from build123d import *

# Parameters (mm, degrees)
SKETCH1_W               = 155
SKETCH1_H               = 163
BOSS_EXTRUDE1_DEPTH     = 10
SKETCH2_R               = 1.5
CUT_EXTRUDE1_DEPTH      = 20
CUT_EXTRUDE2_DEPTH      = 226.153281122
CUT_EXTRUDE2_DEPTH_BACK = 226.153281122
SKETCH3_R               = 1.5


with BuildPart() as part:
    # Sketch1 → Boss-Extrude1 (new body)
    with BuildSketch(Plane(origin=(0, 0, 0), x_dir=(1, 0, 0), z_dir=(0, 1, 0))):
        with Locations((77.5, 81.5)):
            Rectangle(SKETCH1_W, SKETCH1_H)
    extrude(amount=BOSS_EXTRUDE1_DEPTH)

    # Sketch2 → Cut-Extrude1 (cut)
    with BuildSketch(Plane(origin=(0, 0, -163), x_dir=(-1, 0, 0), z_dir=(0, 0, -1))):
        with Locations((-125, 5)):
            Circle(SKETCH2_R)
        with Locations(Location((-30, 5, 0), (0, 0, 180))):
            Circle(SKETCH2_R)
    cut_extrude1 = extrude(amount=-CUT_EXTRUDE1_DEPTH, mode=Mode.SUBTRACT)

    # Mirror1: Cut-Extrude1 across plane
    add(cut_extrude1.mirror(Plane(origin=(0, 0, -81.5), x_dir=(1, 0, 0), z_dir=(0, 0, -1))), mode=Mode.SUBTRACT)

    # Sketch3 → Cut-Extrude2 (cut, two sides: drawn at the far end of the back side and taken through both)
    with BuildSketch(Plane(origin=(155, 0, 0), x_dir=(0, 0, -1), z_dir=(1, 0, 0)).offset(-CUT_EXTRUDE2_DEPTH_BACK)):
        with Locations((35, 5)):
            Circle(SKETCH3_R)
        with Locations(Location((128, 5, 0), (0, 0, 180))):
            Circle(SKETCH3_R)
    extrude(amount=CUT_EXTRUDE2_DEPTH + CUT_EXTRUDE2_DEPTH_BACK, mode=Mode.SUBTRACT)


solid = part.part
The listing builds one solid part. Answer for the finished solid, in the listing's coordinates (mm). Coordinates: 2 decimals unless noted, no trailing zeros. Write each loop counter-clockwise with the first axis right and the second up, starting at its lowest first coordinate (ties: lowest second). Pieces come first, ordered by that corner, then holes. Notation, with made-up numbers: (63.25, 55) - (80.25, 55) arc R20 ccw to (80.25, 61) - close; hole circle Ø3 at (-11.5, -19). An arc over 180 degrees is marked (long way). Return JSON: item names as keys, results as strings.
1. For a pull along X with two mould halves and no side action, classify faces 1 (the face through (76, 5, 0)), 2 (the face through (0, 5, -80)), 3 (the face through (155, 5, -80)) as +X half, -X half, draft (parallel to the pull), parting line (faces both ways), or undercut.
Final values:
{"face 1": "draft", "face 2": "-X half", "face 3": "+X half"}
2. Consider line 1 along Z through (x, y) = (142.5, 4.75); line 2 along Y through (x, z) = (30, -149.5); line 3 along Z through (x, y) = (20, 6.25). Determine where each line is inside the solid, lowest interval first.
Final values:
{"line 1": "-163 to -129.48, -126.52 to -36.48, -33.52 to 0", "line 2": "0 to 3.5, 6.5 to 10", "line 3": "-163 to -128.83, -127.17 to -35.83, -34.17 to 0"}
3. The part is cut by section A-A on y = 5. Determine the outline of the cut face in (x, z), then the cut area to 3 significant figures.
Final values:
{"outline": "(0, -163) - (28.5, -163) - (28.5, -143) - (31.5, -143) - (31.5, -163) - (123.5, -163) - (123.5, -143) - (126.5, -143) - (126.5, -163) - (155, -163) - (155, -129.5) - (0, -129.5) - close; (0, -126.5) - (155, -126.5) - (155, -36.5) - (0, -36.5) - close; (0, -33.5) - (155, -33.5) - (155, 0) - (126.5, 0) - (126.5, -20) - (123.5, -20) - (123.5, 0) - (31.5, 0) - (31.5, -20) - (28.5, -20) - (28.5, 0) - (0, 0) - close", "area": "24,100 mm^2"}
4. Each of these flat-tipped pins is pushed along its axis until it touches: pin 1 Ø2.5 at (y, z) = (5, -128) entering from +X; pin 2 Ø1.5 at (x, y) = (29.5, 4.5) entering from +Z; pin 3 Ø1.5 at (x, y) = (125, 4.5) entering from -Z. Where does it stop, or does it pass through?
Final values:
{"pin 1": "through", "pin 2": "z = -20", "pin 3": "z = -143"}
